Read the model definition and answer for the solid it produces. Units are mm, in the model's axes. Face numbers are marked on the shaded views. A direction names the side the tool comes from. Coordinates: 2 decimals unless noted, no trailing zeros. Loops run counter-clockwise (first coordinate to the right, second up) from the corner with the lowest first, then second, coordinate; pieces in that order, holes last.
Q1. Straight lines are drawn through the part: line 1 (Y direction, x = 7.5, z = 2); line 2 (X direction, y = 26, z = 13.25); line 3 (X direction, y = 24, z = 15.5). For each, find the intervals that lie inside material, in ascending order.
Q2. Section B-B (x = 55) is taken. Give the vertices of the cut face in (y, z).
Q3. Which of the six approach directions +Z, -Z, +X, -X, +Y, -Y give full straight-line access (tool end or side, diameter ignored) to the marked faces 1 and 2?
Q4. Flat-ended cylindrical pins translate along their axes: P1, Ø5, axis at y = 22.5, z = 11.5, coming from the +X side; P2, Ø5, axis at x = 22, y = 16.5, coming from the -Z side; P3, Ø3, axis at x = 57, y = 24, coming from the +Z side. Find the tip coordinate at first contact, or state that the pin passes through.
Q5. Section A-A (z = 23.5) is taken. Give the vertices of the cut face in (x, y), then the cut area to 3 significant figures.
Q6. The mould has two halves that part along Y. Classify the marked faces 3, 4, 5 and 6: pulls with the +Y half, pulls with the -Y half, needs draft (parallel to the pull), parting line crosses it, or undercut.
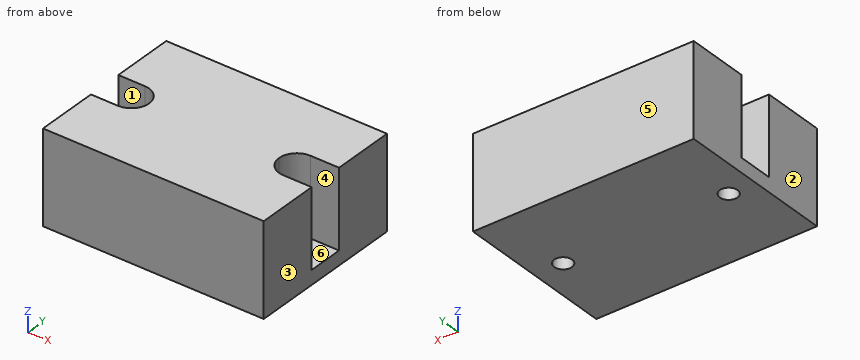
from build123d import *

# Parameters (mm, degrees)
F0_W     = 62
F0_H     = 45
F0_R     = 2.5
F1_DEPTH = 4
F3_DEPTH = 22


with BuildPart() as f1:
    # F0 (on Top) → F1 (new body)
    with BuildSketch(Plane.XY):
        with Locations((31, 22.5)):
            Rectangle(F0_W, F0_H)
        with Locations((7.5, 22.5)):
            Circle(F0_R, mode=Mode.SUBTRACT)
        with Locations((54, 22.5)):
            Circle(F0_R, mode=Mode.SUBTRACT)
    extrude(amount=F1_DEPTH)

    # F2 (on face) → F3 (join)
    with BuildSketch(Plane.XY.offset(4)):
        with BuildLine():
            Line((62, 45), (0, 45))
            Line((0, 45), (0, 27.5))
            Line((0, 27.5), (7.5, 27.5))
            ThreePointArc((7.5, 27.5), (11.035534, 26.035534), (12.5, 22.5))
            ThreePointArc((12.5, 22.5), (11.035534, 18.964466), (7.5, 17.5))
            Line((7.5, 17.5), (0, 17.5))
            Line((0, 17.5), (0, 0))
            Line((0, 0), (62, 0))
            Line((62, 0), (62, 17.5))
            Line((62, 17.5), (54, 17.5))
            ThreePointArc((54, 17.5), (50.464466, 18.964466), (49, 22.5))
            ThreePointArc((49, 22.5), (50.464466, 26.035534), (54, 27.5))
            Line((54, 27.5), (62, 27.5))
            Line((62, 27.5), (62, 45))
        make_face()
    extrude(amount=F3_DEPTH)


solid = f1.part
Numbers:
1. line 1: y = 0 to 20, 25 to 45
1. line 2: x = 11.07 to 50.43
1. line 3: x = 12.27 to 49.23
2. outline: (0, 0) - (20.21, 0) - (20.21, 4) - (17.5, 4) - (17.5, 26) - (0, 26) - close; (24.79, 0) - (45, 0) - (45, 26) - (27.5, 26) - (27.5, 4) - (24.79, 4) - close
3. face 1: +Z, -X
3. face 2: +Z, -Z, -X, +Y, -Y
4. P1: stops at x = 49.67
4. P2: stops at z = 0
4. P3: stops at z = 4
5. outline: (0, 0) - (62, 0) - (62, 17.5) - (54, 17.5) arc R5 cw to (54, 27.5) - (62, 27.5) - (62, 45) - (0, 45) - (0, 27.5) - (7.5, 27.5) arc R5 cw to (7.5, 17.5) - (0, 17.5) - close
5. area: 2,560 mm2
6. face 3: needs draft
6. face 4: undercut
6. face 5: pulls with the +Y half
6. face 6: undercut
